from build123d import *
from OCP.BRepFilletAPI import BRepFilletAPI_MakeChamfer

# Parameters (mm, degrees)
BOSS_EXTRUDE1_DEPTH   = 5
SKETCH1_R             = 2
BOSS_EXTRUDE1_2_DEPTH = 5
BOSS_EXTRUDE1_3_DEPTH = 5
BOSS_EXTRUDE1_4_DEPTH = 5
BOSS_EXTRUDE1_5_DEPTH = 5
SKETCH1_3_W           = 20
SKETCH1_3_H           = 20
BOSS_EXTRUDE2_DEPTH   = 2
SKETCH2_W             = 3.271272918
SKETCH2_H             = 1.91873161
BOSS_EXTRUDE3_DEPTH   = 7
SKETCH2_4_W           = 3.271272918
SKETCH2_4_H           = 1.91873161
BOSS_EXTRUDE4_DEPTH   = 18
CHAMFER1_SIZE         = 1
CHAMFER1_SIZE2        = 5
CHAMFER2_SIZE         = 5
CHAMFER2_SIZE2        = 1
CHAMFER3_SIZE         = 1
CHAMFER3_SIZE2        = 5


with BuildPart() as part:
    # Sketch1 → Boss-Extrude1 (new body)
    with BuildSketch(Plane.XY):
        Polygon((4.925, 10), (-4.925, 10), (-3.125, 8.2), (-5.5, 8.2), (-5.5, 6.560660172), (-2.839339828, 3.9), (2.839339828, 3.9), (5.5, 6.560660172), (5.5, 8.2), (3.125, 8.2), align=None)
    extrude(amount=BOSS_EXTRUDE1_DEPTH)



with BuildPart() as body_2:
    # Sketch1 → Boss-Extrude1 2 (new body)
    with BuildSketch(Plane.XY):
        Circle(SKETCH1_R)
    extrude(amount=BOSS_EXTRUDE1_2_DEPTH)


with BuildPart() as body_3:
    # Sketch1 → Boss-Extrude1 3 (new body)
    with BuildSketch(Plane.XY):
        Polygon((10, -4.925), (10, 4.925), (8.2, 3.125), (8.2, 5.5), (6.560660172, 5.5), (3.9, 2.839339828), (3.9, -2.839339828), (6.560660172, -5.5), (8.2, -5.5), (8.2, -3.125), align=None)
    extrude(amount=BOSS_EXTRUDE1_3_DEPTH)


with BuildPart() as body_4:
    # Sketch1 → Boss-Extrude1 4 (new body)
    with BuildSketch(Plane.XY):
        Polygon((-8.2, 3.125), (-10, 4.925), (-10, -4.925), (-8.2, -3.125), (-8.2, -5.5), (-6.560660172, -5.5), (-3.9, -2.839339828), (-3.9, 2.839339828), (-6.560660172, 5.5), (-8.2, 5.5), align=None)
    extrude(amount=BOSS_EXTRUDE1_4_DEPTH)


with BuildPart() as body_5:
    # Sketch1 → Boss-Extrude1 5 (new body)
    with BuildSketch(Plane.XY):
        Polygon((-3.125, -8.2), (-4.925, -10), (4.925, -10), (3.125, -8.2), (5.5, -8.2), (5.5, -6.560660172), (2.839339828, -3.9), (-2.839339828, -3.9), (-5.5, -6.560660172), (-5.5, -8.2), align=None)
    extrude(amount=BOSS_EXTRUDE1_5_DEPTH)


with BuildPart() as part_1:
    add(part.part)

    add(body_2.part)  # Boss-Extrude2 merges body 2

    add(body_3.part)  # Boss-Extrude2 merges body 3

    add(body_4.part)  # Boss-Extrude2 merges body 4

    add(body_5.part)  # Boss-Extrude2 merges body 5
    # Sketch1_3 → Boss-Extrude2 (add)
    with BuildSketch(Plane.XY):
        Rectangle(SKETCH1_3_W, SKETCH1_3_H)
    extrude(amount=-BOSS_EXTRUDE2_DEPTH)

    # Sketch2 → Boss-Extrude3 (add)
    with BuildSketch(Plane.XY.offset(5)):
        Polygon((-5.5, 11.91873161), (-1.635636459, 11.91873161), (1.635636459, 11.91873161), (5.5, 11.91873161), (5.5, 13.01873161), (2.6, 15.91873161), (0, 15.91873161), (-2.6, 15.91873161), (-5.5, 13.01873161), align=None)
        with Locations((0, 10.959365805)):
            Rectangle(SKETCH2_W, SKETCH2_H)
    extrude(amount=-BOSS_EXTRUDE3_DEPTH)

    # Sketch2_4 → Boss-Extrude4 (add)
    with BuildSketch(Plane.XY.offset(5)):
        Polygon((-5.5, 8.08126839), (-5.5, 6.98126839), (-2.6, 4.08126839), (0, 4.08126839), (2.6, 4.08126839), (5.5, 6.98126839), (5.5, 8.08126839), (1.635636459, 8.08126839), (-1.635636459, 8.08126839), align=None)
        with Locations((0, 9.040634195)):
            Rectangle(SKETCH2_4_W, SKETCH2_4_H)
        with Locations((0, 10.959365805)):
            Rectangle(SKETCH2_4_W, SKETCH2_4_H)
        Polygon((-5.5, 11.91873161), (-1.635636459, 11.91873161), (1.635636459, 11.91873161), (5.5, 11.91873161), (5.5, 13.01873161), (2.6, 15.91873161), (0, 15.91873161), (-2.6, 15.91873161), (-5.5, 13.01873161), align=None)
    extrude(amount=BOSS_EXTRUDE4_DEPTH)

    # Chamfer1
    chamfer1_edges = [part_1.edges().sort_by_distance(p)[0] for p in [
        (4.05, 14.46873161, 23),
        (0, 15.91873161, 23),
        (-4.05, 14.46873161, 23),
    ]]
    chamfer1_side = [part_1.faces().sort_by_distance(p)[0] for p in [
        (0, 10, 23),
    ]]
    chamfer(chamfer1_edges, length=CHAMFER1_SIZE, length2=CHAMFER1_SIZE2, reference=chamfer1_side[0])

    # Chamfer2: one chamfer whose edges measure the first distance from different faces: ONE call of the kernel's chamfer builder (chamfer() names one face for all edges)
    chamfer2_edges_1 = [part_1.edges().sort_by_distance(p)[0] for p in [
        (4.05, 14.46873161, -2),
    ]]
    chamfer2_side_1 = [part_1.faces().sort_by_distance(p)[0] for p in [
        (4.05, 14.46873161, 8),
    ]]
    chamfer2_edges_2 = [part_1.edges().sort_by_distance(p)[0] for p in [
        (0, 15.91873161, -2),
    ]]
    chamfer2_side_2 = [part_1.faces().sort_by_distance(p)[0] for p in [
        (0, 15.91873161, 8),
    ]]
    chamfer2_edges_3 = [part_1.edges().sort_by_distance(p)[0] for p in [
        (-4.05, 14.46873161, -2),
    ]]
    chamfer2_side_3 = [part_1.faces().sort_by_distance(p)[0] for p in [
        (-4.05, 14.46873161, 8),
    ]]
    chamfer2 = BRepFilletAPI_MakeChamfer(part_1.part.solid().wrapped)
    for e in chamfer2_edges_1:
        chamfer2.Add(CHAMFER2_SIZE, CHAMFER2_SIZE2, e.wrapped, chamfer2_side_1[0].wrapped)  # the first distance lies on this face
    for e in chamfer2_edges_2:
        chamfer2.Add(CHAMFER2_SIZE, CHAMFER2_SIZE2, e.wrapped, chamfer2_side_2[0].wrapped)  # the first distance lies on this face
    for e in chamfer2_edges_3:
        chamfer2.Add(CHAMFER2_SIZE, CHAMFER2_SIZE2, e.wrapped, chamfer2_side_3[0].wrapped)  # the first distance lies on this face
    add(Compound.cast(chamfer2.Shape()), mode=Mode.REPLACE)

    # Chamfer3
    chamfer3_edges = [part_1.edges().sort_by_distance(p)[0] for p in [
        (4.05, 5.53126839, 23),
        (0, 4.08126839, 23),
        (-4.05, 5.53126839, 23),
    ]]
    chamfer3_side = [part_1.faces().sort_by_distance(p)[0] for p in [
        (0, 9.15065978, 23),
    ]]
    chamfer(chamfer3_edges, length=CHAMFER3_SIZE, length2=CHAMFER3_SIZE2, reference=chamfer3_side[0])


solid = part_1.part
Here's how the part is built. I have some questions about the finished solid (model axes, mm). A direction names the side the tool comes from. Coordinates: 2 decimals unless noted, no trailing zeros. Write each loop counter-clockwise with the first axis right and the second up, starting at its lowest first coordinate (ties: lowest second). Pieces come first, ordered by that corner, then holes.
1) Which directions (+Z, -Z, +X, -X, +Y, -Y) give clear straight access to the entire face, cutting with the end or side of a thin tool? Please do faces 5 (the face through (-7, -5.5, 2)), 6 (the face through (-4, 11.919, 10)), 7 (the face through (-3, 9, 5)), 8 (the face through (7, -5.5, 2)), 9 (the face through (0, -3.9, 2)).
Filled in:
face 5: +Z, -X, -Y
face 6: +Z, -Z, -X
face 7: +Z, -X
face 8: +Z, +X, -Y
face 9: +Z
2) If we section it at C-C (y = 2.5): List the corners of the cut face in (x, z) for me, plus the area to 3 significant figures.
Filled in:
outline: (-10, -2) - (10, -2) - (10, 5) - (3.9, 5) - (3.9, 0) - (-3.9, 0) - (-3.9, 5) - (-10, 5) - close
area: 101 mm2
3) If we section it at A-A (z = 17): List the corners of the cut face in (x, y) for me.
Filled in:
outline: (-5.5, 6.98) - (-2.6, 4.08) - (2.6, 4.08) - (5.5, 6.98) - (5.5, 8.08) - (1.64, 8.08) - (1.64, 11.92) - (5.5, 11.92) - (5.5, 13.02) - (2.6, 15.92) - (-2.6, 15.92) - (-5.5, 13.02) - (-5.5, 11.92) - (-1.64, 11.92) - (-1.64, 8.08) - (-5.5, 8.08) - close
4) If we section it at D-D (y = -3.5): List the corners of the cut face in (x, z) for me (3 decimals).
Filled in:
outline: (-10, -2) - (10, -2) - (10, 5) - (8.575, 5) - (8.575, 0) - (8.2, 0) - (8.2, 5) - (4.561, 5) - (4.561, 0) - (-4.561, 0) - (-4.561, 5) - (-8.2, 5) - (-8.2, 0) - (-8.575, 0) - (-8.575, 5) - (-10, 5) - close
5) I'm going to push flat-ended pins straight in: pin 1 (3 mm diameter, centred on y = 11, z = 12, fed in from -X); pin 2 (1 mm diameter, centred on x = -3.5, y = 9, fed in from +Z); pin 3 (2.5 mm diameter, centred on x = -5, z = 1.5, fed in from -Y); pin 4 (5.5 mm diameter, centred on x = 0.5, z = 12.5, fed in from -Y). Where does each tip first touch, or does it pass through?
Filled in:
pin 1: stops at x = -5.5
pin 2: stops at z = 5
pin 3: stops at y = -10
pin 4: stops at y = 4.08
6) If I drill on line 1 (Y direction, x = 6.25, z = 4); line 2 (Z direction, x = 8.75, y = 9.75); line 3 (Z direction, x = -1.25, y = -8), over which ranges is the centre line in solid material (lowest first)?
Filled in:
line 1: y = -5.19 to 5.19
line 2: z = -2 to 0
line 3: z = -2 to 5
7) If we section it at B-B (x = 0): List the corners of the cut face in (y, z) for me.
Filled in:
outline: (-10, -2) - (14.92, -2) - (15.92, 3) - (15.92, 18) - (14.92, 23) - (5.08, 23) - (4.08, 18) - (4.08, 5) - (3.9, 5) - (3.9, 0) - (2, 0) - (2, 5) - (-2, 5) - (-2, 0) - (-3.9, 0) - (-3.9, 5) - (-10, 5) - close
8) Thinking about a two-plate mould opening in Y: for faces 1 (the face through (4.07, 14.45, 10.4)), 2 (the face through (3.952, 6.131, 20.465)), 3 (the face through (5.5, 12.5, 10.3)), 4 (the face through (4.19, -5.25, 2.46)), which applies, +Y half, -Y half, draft (parallel to the pull), parting line (faces both ways), or undercut?
Filled in:
face 1: +Y half
face 2: -Y half
face 3: draft
face 4: undercut
